Input: part model. Units: mm. Frame: model coordinates. Face numbers are marked on the shaded views. Round coordinates to 2 decimals unless told otherwise and drop trailing zeros. Loops run counter-clockwise (first coordinate to the right, second up) from the corner with the lowest first, then second, coordinate; pieces in that order, holes last. Notation, with made-up numbers: M 75.5,70 L 85.5,70 A8 cw 85.5,77 Z; hole C -1,1.25 d11. An arc over 180 degrees is marked long. Put each result on its own line as item: value. Start each with the question number.
1) Pin query (flat end, axial travel): pin 1 (6 mm diameter, centred on x = -1.5, z = -20, fed in from -Y); pin 2 (4.5 mm diameter, centred on x = 0, y = -1, fed in from -Z); pin 3 (2 mm diameter, centred on x = 5.5, z = -11.5, fed in from -Y); pin 4 (6 mm diameter, centred on x = 4.5, z = -3.5, fed in from -Y). Return the tip coordinate at first contact, or that it passes through.
2) Draft query along X for the marked faces 1, 2 and 3. Return one class per face: +X half, -X half, draft (parallel to the pull), parting line (faces both ways), or undercut.
3) Section B-B on y = 0. Output: boundary loops of the cut face in (x, z).
4) Section D-D on z = -4. Output: boundary loops of the cut face in (x, y).
5) Section A-A on x = 0. Output: boundary loops of the cut face in (y, z), plus the area to 3 significant figures.
6) Section C-C on z = -16.5. Output: boundary loops of the cut face in (x, y).
7) Line query: probe 1 along Y at (x, z) = (0, -8.25); probe 2 along Z at (x, y) = (0, 6.3); probe 3 along Y at (x, z) = (-3.5, -15). Output: solid intervals per line, ascending.
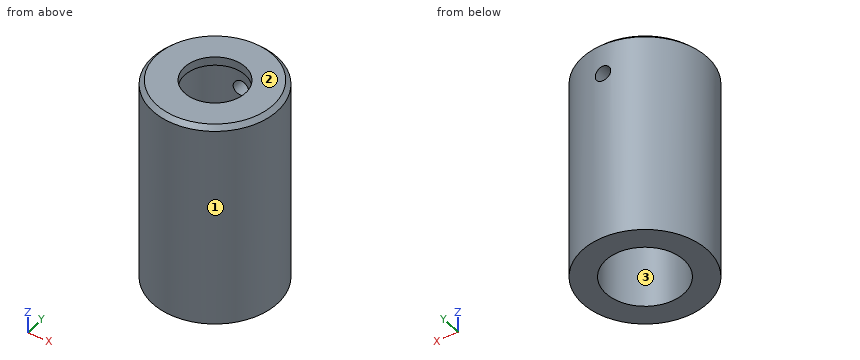
from build123d import *

# Parameters (mm, degrees)
F_2_56_TAPPED_HOLE2_REACH  = 16.5
F_2_56_TAPPED_HOLE2_BORE_R = 0.889
CHAMFER1_SIZE              = 0.5


with BuildPart() as part:
    # Sketch1 → Revolve1 (revolve)
    with BuildSketch(Plane(origin=(0, 0, 0), x_dir=(0, 0, -1), z_dir=(1, 0, 0)), mode=Mode.PRIVATE) as revolve1_sk:
        Polygon((0, 7.25), (0, 3.53), (1, 3.53), (1, 4.53), (24, 4.53), (24, 7.25), align=None)
    revolve(revolve1_sk.sketch.rotate(Axis((0, 0, 0), (0, 0, 1)), 90), axis=Axis((0, 0, 0), (0, 0, 1)))  # turned: the seam where the file's is

    # #2-56 Tapped Hole2 bore (on position points) → #2-56 Tapped Hole2 (cut, up to next)
    with BuildSketch(Plane(origin=(0, 7.25, -4), x_dir=(1, 0, 0), z_dir=(0, 1, 0)), mode=Mode.PRIVATE) as f_2_56_tapped_hole2_sk1:
        Circle(F_2_56_TAPPED_HOLE2_BORE_R)
    f_2_56_tapped_hole2_tool1 = extrude(f_2_56_tapped_hole2_sk1.sketch, amount=-F_2_56_TAPPED_HOLE2_REACH, mode=Mode.PRIVATE) & part.part
    add(f_2_56_tapped_hole2_tool1.solids().sort_by_distance((0, 7.25, -4))[0], mode=Mode.SUBTRACT)

    # Chamfer1
    chamfer1_edges = [part.edges().sort_by_distance(p)[0] for p in [
        (7.25, 0, 0),
    ]]
    chamfer(chamfer1_edges, length=CHAMFER1_SIZE)


solid = part.part
Geometry results:
1. pin 1: stops at y = -7.25
1. pin 2: passes through
1. pin 3: stops at y = -5.68
1. pin 4: stops at y = -7.09
2. face 1: parting line
2. face 2: draft
2. face 3: undercut
3. outline: M -7.25,-24 L -4.53,-24 L -4.53,-1 L -3.53,-1 L -3.53,0 L -6.75,0 L -7.25,-0.5 Z; M 3.53,-1 L 4.53,-1 L 4.53,-24 L 7.25,-24 L 7.25,-0.5 L 6.75,0 L 3.53,0 Z
4. outline: M -0.89,4.44 L -0.89,7.2 A7.25 ccw long 0.89,7.2 L 0.89,4.44 A4.53 cw long Z
5. outline: M -7.25,-24 L -4.53,-24 L -4.53,-1 L -3.53,-1 L -3.53,0 L -6.75,0 L -7.25,-0.5 Z; M 3.53,-1 L 4.53,-1 L 4.53,-3.11 L 7.25,-3.11 L 7.25,-0.5 L 6.75,0 L 3.53,0 Z; M 4.53,-24 L 7.25,-24 L 7.25,-4.89 L 4.53,-4.89 Z
5. area: 127 mm²
6. outline: C 0,0 d14.5; hole C 0,0 d9.06
7. probe 1: y = -7.25 to -4.53, 4.53 to 7.25
7. probe 2: z = -24 to -4.89, -3.11 to 0
7. probe 3: y = -6.35 to -2.88, 2.88 to 6.35
